from build123d import *

# Parameters (mm, degrees)
BOSS_EXTRUDE1_DEPTH = 2
CHAMFER1_SIZE       = 8
BOSS_EXTRUDE2_DEPTH = 1.5
SKETCH4_W           = 99.768826376
SKETCH4_H           = 91.588754032
CUT_EXTRUDE1_DEPTH  = 2
SKETCH5_R           = 2.5
CUT_EXTRUDE2_DEPTH  = 2
SKETCH6_R           = 3.5
CUT_EXTRUDE3_DEPTH  = 1
CHAMFER2_SIZE       = 1


with BuildPart() as part:
    # Sketch1 → Boss-Extrude1 (new body)
    with BuildSketch(Plane(origin=(0, 0, 0), x_dir=(1, 0, 0), z_dir=(0, 1, 0))):
        Polygon((-1.782487159, -28.34466675), (33.85093234, -28.34466675), (33.85093234, 27.435918205), (-31.480603593, 27.435918205), (-31.480603593, 2.026433414), (-44.933505709, 2.026433414), (-44.933505709, -41.124585136), (-1.782487159, -41.124585136), align=None)
    extrude(amount=BOSS_EXTRUDE1_DEPTH)

    # Chamfer1
    chamfer1_edges = [part.edges().sort_by_distance(p)[0] for p in [
        (-44.933505709, 1, 41.124585136),
    ]]
    chamfer(chamfer1_edges, length=CHAMFER1_SIZE)

    # Sketch3 → Boss-Extrude2 (add)
    with BuildSketch(Plane(origin=(0, 2, 0), x_dir=(1, 0, 0), z_dir=(0, 1, 0))):
        Polygon((-29.480603593, 25.435918205), (31.85093234, 25.435918205), (31.85093234, -26.34466675), (-3.782487159, -26.34466675), (-3.782487159, -39.124585136), (-36.105078585, -39.124585136), (-42.933505709, -32.296158012), (-42.933505709, 0.026433414), (-29.480603593, 0.026433414), align=None)
    extrude(amount=BOSS_EXTRUDE2_DEPTH)

    # Sketch4 → Cut-Extrude1 (cut)
    with BuildSketch(Plane.XZ):
        Rectangle(SKETCH4_W, SKETCH4_H)
    extrude(amount=-CUT_EXTRUDE1_DEPTH, mode=Mode.SUBTRACT)

    # Sketch5 → Cut-Extrude2 (cut)
    with BuildSketch(Plane(origin=(0, 3.5, 0), x_dir=(1, 0, 0), z_dir=(0, 1, 0))):
        with Locations(Location((-18.814835626, 18.545625727, 0), (0, 0, 270))):
            Circle(SKETCH5_R)
        with Locations(Location((21.185164374, 18.545625727, 0), (0, 0, 270))):
            Circle(SKETCH5_R)
        with Locations(Location((21.185164374, -19.454374273, 0), (0, 0, 270))):
            Circle(SKETCH5_R)
        with Locations(Location((-29.854835626, -26.529137879, 0), (0, 0, 270))):
            Circle(SKETCH5_R)
    extrude(amount=-CUT_EXTRUDE2_DEPTH, mode=Mode.SUBTRACT)

    # Sketch6 → Cut-Extrude3 (cut)
    with BuildSketch(Plane.XZ.offset(-2)):
        with Locations(Location((-29.854835626, 26.529137879, 0), (0, 0, 270))):
            Circle(SKETCH6_R)
        with Locations(Location((21.185164374, 19.454374273, 0), (0, 0, 270))):
            Circle(SKETCH6_R)
        with Locations(Location((-18.814835626, -18.545625727, 0), (0, 0, 270))):
            Circle(SKETCH6_R)
        with Locations(Location((21.185164374, -18.545625727, 0), (0, 0, 270))):
            Circle(SKETCH6_R)
    extrude(amount=-CUT_EXTRUDE3_DEPTH, mode=Mode.SUBTRACT)

    # Chamfer2
    chamfer2_edges = [part.edges().sort_by_distance(p)[0] for p in [
        (-29.480603593, 2, -12.731175809),
        (-36.207054651, 2, -0.026433414),
        (-42.933505709, 2, 16.134862299),
        (-39.519292147, 2, 35.710371574),
        (-19.943782872, 2, 39.124585136),
        (-3.782487159, 2, 32.734625943),
        (14.034222591, 2, 26.34466675),
        (31.85093234, 2, 0.454374273),
        (1.185164374, 2, -25.435918205),
    ]]
    chamfer(chamfer2_edges, length=CHAMFER2_SIZE)


solid = part.part
Source: CAD feature listing. Evaluate the final solid. Frame: model axes, mm. A direction names the side the tool comes from. Round coordinates to 2 decimals unless told otherwise and drop trailing zeros. Order: outer loops, then holes, each group sorted by start corner. A loop starts at its lowest first (then second) coordinate and runs counter-clockwise, first axis right, second up. Notation, with made-up numbers: (54.5, -33) -> (81.5, -33) arc R29 cw to (81.5, -13) -> close; hole circle Ø7 at (2, 10.5). An arc over 180 degrees is marked (long way). Answer as CSV lines item,"result".
Item 1: Section B-B, the plane y = 2.3. Return loops of the section in (x, z), plus the area to 3 significant figures.
A:
outline,"(-42.23, 0.67) -> (-28.78, 0.67) -> (-28.78, -24.74) -> (31.15, -24.74) -> (31.15, 25.64) -> (-4.48, 25.64) -> (-4.48, 38.42) -> (-35.82, 38.42) -> (-42.23, 32.01) -> close; hole circle Ø7 at (-29.85, 26.53); hole circle Ø7 at (-18.81, -18.55); hole circle Ø7 at (21.19, -18.55); hole circle Ø7 at (21.19, 19.45)"
area,"3,660 mm²"
Item 2: Reachability of faces 4 (the face through (19.664, 3.254, -20.53)), 5 (the face through (-33.27, 2.49, 27.29)) from +Z, -Z, +X, -X, +Y, -Y: full face, straight path, thin tool, end or side. Return the list, or none.
A:
face 4,"+Y, -Y"
face 5,"-Y"
Item 3: Section A-A, the plane x = 10. Return loops of the section in (y, z), plus the area to 3 significant figures.
A:
outline,"(2, -24.44) -> (3, -25.44) -> (3.5, -25.44) -> (3.5, 26.34) -> (3, 26.34) -> (2, 25.34) -> close"
area,"76.7 mm²"
Item 4: Pin query (flat end, axial travel): pin 1 Ø2 at (x, z) = (20.5, -19) entering from -Y; pin 2 Ø9 at (x, z) = (21.19, -18.55) entering from -Y; pin 3 Ø0.6 at (y, z) = (3.5, 33) entering from +X; pin 4 Ø3.5 at (x, z) = (-19, -20) entering from -Y. Return the tip coordinate at first contact, or that it passes through.
A:
pin 1,"through"
pin 2,"y = 2"
pin 3,"x = -3.78"
pin 4,"y = 3"
Item 5: Pull-direction query (Z, two-part tool) for faces 1 (the face through (19.664, 3.254, 17.47)), 2 (the face through (-6, 2, 7)), 3 (the face through (-39.47, 3.25, 35.76)); classes: pulls with the +Z half, pulls with the -Z half, needs draft (parallel to the pull), parting line crosses it, or undercut.
A:
face 1,"undercut"
face 2,"needs draft"
face 3,"pulls with the +Z half"
Item 6: Section C-C, the plane z = -9.5. Return loops of the section in (x, y), plus the area to 3 significant figures.
A:
outline,"(-29.48, 3) -> (-28.48, 2) -> (30.85, 2) -> (31.85, 3) -> (31.85, 3.5) -> (-29.48, 3.5) -> close"
area,"91.0 mm²"
Item 7: Line query: L1, parallel to Z at x = 21.5, y = 2.2; L2, parallel to X at y = 2.5, z = 25.5; L3, parallel to Z at x = 4, y = 3.25. Output: solid intervals per line, ascending.
A:
L1,"-24.64 to -22.03, -15.06 to 15.97, 22.94 to 25.54"
L2,"-42.43 to -33.2, -26.51 to 31.35"
L3,"-25.44 to 26.34"
